The listing builds one solid part. Answer for the finished solid, in the listing's coordinates (mm). A direction names the side the tool comes from. Give positions to 0.01 mm unless a question says otherwise; leave off trailing zeros. Loops run counter-clockwise (first coordinate to the right, second up) from the corner with the lowest first, then second, coordinate; pieces in that order, holes last. Notation, with made-up numbers: (48.5, -40) - (96.5, -40) arc R26 cw to (96.5, -24) - close; hole circle Ø7 at (-7.5, -9.75). An arc over 180 degrees is marked (long way). Write each question's results on one line, items separated by ' | '.
from build123d import *

# Parameters (mm, degrees)
SKETCH1_R           = 7
BOSS_EXTRUDE1_DEPTH = 43
CUT_EXTRUDE1_DEPTH  = 42


with BuildPart() as part:
    # Sketch1 → Boss-Extrude1 (new body)
    with BuildSketch(Plane.XY):
        with BuildLine():
            Line((-14, -7), (-14, 11))
            Line((-14, 11), (-7, 18))
            Line((-7, 18), (0, 18))
            Line((0, 18), (18.243084988, 14.783251905))
            ThreePointArc((18.243084988, 14.783251905), (29.574972961, 16.276069151), (38, 24))
            Line((38, 24), (62, 24))
            Line((62, 24), (67, 19))
            Line((67, 19), (67, 0))
            Line((67, 0), (38, -33))
            Line((38, -33), (32.788067397, -33))
            ThreePointArc((32.788067397, -33), (28.3490952, -26.115672061), (26.012264997, -18.264705882))
            ThreePointArc((26.012264997, -18.264705882), (24.331862036, -15.213413768), (21.066626255, -14))
            Line((21.066626255, -14), (-7, -14))
            Line((-7, -14), (-14, -7))
        make_face()
        Circle(SKETCH1_R, mode=Mode.SUBTRACT)
    extrude(amount=BOSS_EXTRUDE1_DEPTH)

    # Sketch2 → Cut-Extrude1 (cut)
    with BuildSketch(Plane.XY.offset(43)):
        with BuildLine():
            Line((8, 0), (38, 0))
            Line((38, 0), (38, -31.485111542))
            Line((38, -31.485111542), (37.547522264, -32))
            Line((37.547522264, -32), (33.249359107, -32))
            ThreePointArc((33.249359107, -32), (29.163792236, -25.491599052), (27.001392745, -18.117647059))
            ThreePointArc((27.001392745, -18.117647059), (24.984909193, -14.456096521), (21.066626255, -13))
            Line((21.066626255, -13), (-6.585786438, -13))
            Line((-6.585786438, -13), (-13, -6.585786438))
            Line((-13, -6.585786438), (-13, 0))
            Line((-13, 0), (-8, 0))
            ThreePointArc((-8, 0), (0, -8), (8, 0))
        make_face()
    extrude(amount=-CUT_EXTRUDE1_DEPTH, mode=Mode.SUBTRACT)


solid = part.part
Item 1: Flat-ended cylindrical pins translate along their axes: P1, Ø5.5, axis at x = -4.5, z = 13.5, coming from the +Y side; P2, Ø1.5, axis at x = -10, z = 20, coming from the -Y side; P3, Ø15, axis at x = 22, z = 15, coming from the -Y side; P4, Ø3, axis at x = 22, y = -16, coming from the -Z side. Find the tip coordinate at first contact, or state that the pin passes through.
Values found:
P1: stops at y = 18 | P2: stops at y = -11.75 | P3: stops at y = -28.36 | P4: passes through
Item 2: For faces 1 (the face through (-4, 18, 21)), 2 (the face through (52.7, -16.27, 21.2)), 3 (the face through (7, -14, 21)), 4 (the face through (8.994, 16.414, 21.199)), 5 (the face through (-11, 0, 22)), determine the directions among +Z, -Z, +X, -X, +Y, -Y from which every point of the face is accessible in a straight line to the end or side of a thin tool.
Values found:
face 1: +Z, -Z, -X, +Y | face 2: +Z, -Z, +X, -Y | face 3: +Z, -Z, -X, -Y | face 4: +Z, -Z, +Y | face 5: +Z
Item 3: A cutting plane is placed at C-C, the plane x = -5. Determine the outline of the cut face in (y, z) (3 decimals), plus the area to 3 significant figures.
Values found:
outline: (-14, 0) - (-4.899, 0) - (-4.899, 43) - (-6.245, 43) - (-6.245, 1) - (-13, 1) - (-13, 43) - (-14, 43) - close; (4.899, 0) - (18, 0) - (18, 43) - (4.899, 43) - close | area: 671 mm²
Item 4: A cutting plane is placed at D-D, the plane y = -21.5. Determine the outline of the cut face in (x, z).
Values found:
outline: (26.68, 0) - (48.11, 0) - (48.11, 43) - (38, 43) - (38, 1) - (27.72, 1) - (27.72, 43) - (26.68, 43) - close
Item 5: A cutting plane is placed at A-A, the plane z = 29.5. Determine the outline of the cut face in (x, y).
Values found:
outline: (-14, -7) - (-7, -14) - (21.07, -14) arc R5 cw to (26.01, -18.26) arc R29 ccw to (32.79, -33) - (38, -33) - (67, 0) - (67, 19) - (62, 24) - (38, 24) arc R19 cw to (18.24, 14.78) - (0, 18) - (-7, 18) - (-14, 11) - close; hole (-13, -6.59) - (-6.59, -13) - (21.07, -13) arc R6 cw to (27, -18.12) arc R28 ccw to (33.25, -32) - (37.55, -32) - (38, -31.49) - (38, 0) - (8, 0) arc R8 cw to (-8, 0) - (-13, 0) - close; hole circle Ø14 at (0, 0)
Item 6: Find the intervals of material crossed by line 1 along Y through (x, z) = (0, 33.5); line 2 along X through (y, z) = (-21.5, 22); line 3 along X through (y, z) = (-12.5, 33), in increasing order. Write a range as [from, to].
Values found:
line 1: y = [-14, -13], [-8, -7], [7, 18] | line 2: x = [26.68, 27.72], [38, 48.11] | line 3: x = [-8.5, -7.09], [38, 56.02]
Item 7: A cutting plane is placed at B-B, the plane y = -2.5. Determine the outline of the cut face in (x, z).
Values found:
outline: (-14, 0) - (-6.54, 0) - (-6.54, 43) - (-7.6, 43) - (-7.6, 1) - (-13, 1) - (-13, 43) - (-14, 43) - close; (6.54, 0) - (64.8, 0) - (64.8, 43) - (38, 43) - (38, 1) - (7.6, 1) - (7.6, 43) - (6.54, 43) - close
Item 8: For a pull along Y with two mould halves and no side action, classify faces 6 (the face through (27, 2, 0)), 7 (the face through (35, -33, 21)), 8 (the face through (35, -32, 22)) as released by +Y, released by -Y, zero draft, split by the parting line, or undercut.
Values found:
face 6: zero draft | face 7: released by -Y | face 8: undercut
